Could you check a few things on this model? Use its own coordinates, in mm. A direction names the side the tool comes from. Coordinates: 2 decimals unless noted, no trailing zeros. Loops run counter-clockwise (first coordinate to the right, second up) from the corner with the lowest first, then second, coordinate; pieces in that order, holes last.
1) Imagine slicing it at B-B on z = 42.5. Please give me the cut outline in (x, y), plus the area to 3 significant figures.
2) Imagine slicing it at C-C on z = 30. Please give me the cut outline in (x, y), plus the area to 3 significant figures.
3) Will these pins go through, and if not, where does the flat tip stop? P1, Ø6, axis at x = 0.5, y = -3, coming from the -Z side; P2, Ø2.5, axis at x = 0.5, z = 46, coming from the +Y side; P3, Ø1.6, axis at x = 1, z = 41.5, coming from the -Y side; P4, Ø6, axis at y = 3, z = 19.5, coming from the -X side.
4) Thinking about a two-plate mould opening in Z: for faces 5 (the face through (0, -5, 33.916)), 6 (the face through (-0.96, 4.34, 1.16)), 7 (the face through (-5, 2, 15.803)), 8 (the face through (0, -4.762, 46)), which applies, released by +Z, released by -Z, zero draft, split by the parting line, or undercut?
5) If I drill on line 1 along Z through (x, y) = (5.5, -3.75); line 2 along Z through (x, y) = (4.25, -4); line 3 along Y through (x, z) = (-0.5, 55.5), over which ranges is the centre line in solid material (lowest first)?
6) For faces 1 (the face through (-4.144, 2.348, 8.567)), 2 (the face through (4.144, -2.348, 8.567)), 3 (the face through (0, 4.762, 9)), 4 (the face through (-6, 0, 24)), which set-ups out of +Z, -Z, +X, -X, +Y, -Y let a thin tool reach every point of the face, with its end or its side?
Autodesk Inventor part; units mm, degrees
ref_plane "YZ Plane" through (0, 0, 0) normal (1, 0, 0) x (0, 1, 0)
ref_plane "XZ Plane" through (0, 0, 0) normal (0, 1, 0) x (-1, 0, 0)
ref_plane "XY Plane" through (0, 0, 0) normal (0, 0, 1) x (1, 0, 0)
sketch "Sketch1" plane through (0, 0, 0) normal (0, 0, 1) x (1, 0, 0)
  circle A0 centre (0, 0) radius 4.7625
  dimension "d0" = 9.525
extrude "Extrusion1" add sketch "Sketch1" along normal blind 0.7937
sketch "Sketch2" plane through (0, 0, 0.7937) normal (0, 0, 1) x (1, 0, 0)
  circle A0 centre (0, 0) radius 4.7625
  circle A1 centre (0, 0) radius 4.445
  dimension "d3" = 8.89
extrude "Extrusion2" add sketch "Sketch2" along normal blind 0.7366 contours A1
sketch "Sketch3" plane through (0, 0, 1.5304) normal (0, 0, 1) x (1, 0, 0)
  circle A0 centre (0, 0) radius 4.445
  line L0 (5.4993, 0) -> (2.7496, -4.7625)
  line L1 (2.7496, -4.7625) -> (-2.7496, -4.7625)
  line L2 (-2.7496, -4.7625) -> (-5.4993, 0)
  line L3 (-5.4993, 0) -> (-2.7496, 4.7625)
  line L4 (-2.7496, 4.7625) -> (2.7496, 4.7625)
  line L5 (2.7496, 4.7625) -> (5.4993, 0)
  dimension "d6" = 9.525
extrude "Extrusion3" add sketch "Sketch3" along normal blind 14.273 contours A0 | L0 L1 L2 L3 L4 L5
sketch "Sketch4" plane through (0, 0, 15.8034) normal (0, 0, 1) x (1, 0, 0)
  circle A0 centre (0, 0) radius 5.5563
  dimension "d9" = 11.1125
extrude "Extrusion4" add sketch "Sketch4" along normal blind 4.9219
sketch "Sketch8" plane through (0, 0, 20.7252) normal (0, 0, 1) x (1, 0, 0)
  circle A0 centre (0, 0) radius 5.5562
  circle A1 centre (0, 0) radius 6
  dimension "d24" = 12
extrude "Extrusion8" add sketch "Sketch8" along normal blind 6 contours A0 | A1
sketch "Sketch5" plane through (0, 0, 26.7252) normal (0, 0, 1) x (1, 0, 0)
  circle A0 centre (0, 0) radius 7.1437
  dimension "d12" = 14.2875
extrude "Extrusion5" add sketch "Sketch5" along normal blind 1.1906
sketch "Sketch6" plane through (0, 0, 27.9159) normal (0, 0, 1) x (1, 0, 0)
  circle A0 centre (0, 0) radius 7.1437
  circle A1 centre (0, 0) radius 6
  dimension "d15" = 12
extrude "Extrusion6" add sketch "Sketch6" along normal blind 6 contours A1
sketch "Sketch7" plane through (0, 0, 33.9159) normal (0, 0, 1) x (1, 0, 0)
  circle A0 centre (0, 0) radius 6
  line L0 (2.7496, 4.7625) -> (5.4993, 0)
  line L1 (5.4993, 0) -> (2.7496, -4.7625)
  line L2 (2.7496, -4.7625) -> (-2.7496, -4.7625)
  line L3 (-2.7496, -4.7625) -> (-5.4993, 0)
  line L4 (-5.4993, 0) -> (-2.7496, 4.7625)
  line L5 (-2.7496, 4.7625) -> (2.7496, 4.7625)
  dimension "d18" = 9.525
extrude "Extrusion7" add sketch "Sketch7" along normal blind 25.4 contours L0 L1 L2 L3 L4 L5
chamfer "Chamfer1" distance 0.3969 angle 45 1 edges at (-4.7625, 0, 0)
properties part number "Module Top Shaft" material "Aluminum 6061"
Filled in:
1. outline: (-5.5, 0) - (-2.75, -4.76) - (2.75, -4.76) - (5.5, 0) - (2.75, 4.76) - (-2.75, 4.76) - close
1. area: 78.6 mm2
2. outline: circle Ø12 at (0, 0)
2. area: 113 mm2
3. P1: stops at z = 0
3. P2: stops at y = 4.76
3. P3: stops at y = -4.76
3. P4: stops at x = -5.99
4. face 5: released by +Z
4. face 6: undercut
4. face 7: released by -Z
4. face 8: zero draft
5. line 1: z = 26.73 to 27.92
5. line 2: z = 20.73 to 33.92
5. line 3: y = -4.76 to 4.76
6. face 1: -Z, -X, +Y
6. face 2: -Z, +X, -Y
6. face 3: -Z, +X, -X, +Y
6. face 4: -Z
